Source: CAD feature listing. Evaluate the final solid. Frame: model axes, mm. A direction names the side the tool comes from. Give positions to 0.01 mm unless a question says otherwise; leave off trailing zeros. Order: outer loops, then holes, each group sorted by start corner. A loop starts at its lowest first (then second) coordinate and runs counter-clockwise, first axis right, second up.
1) Section B-B, the plane x = -20. Return loops of the section in (y, z), plus the area to 3 significant figures.
2) Section C-C, the plane y = 21. Return loops of the section in (x, z).
3) Section A-A, the plane z = 0. Return loops of the section in (x, y), plus the area to 3 significant figures.
4) Material intervals for line 1 (X direction, y = 65, z = 25.5); line 2 (Z direction, x = -20, y = 23); line 3 (Y direction, x = -32, z = -27) (3 decimals), sorted ascending.
5) First-contact query: P1, Ø10, axis at y = 13.5, z = 15.5, coming from the +X side; P2, Ø7, axis at x = 30.5, z = 2, coming from the +Y side; P3, Ø20.5, axis at x = 35, z = 0, coming from the +Y side. Flat tips, straight axial feed; report the tip coordinate or a pass-through.
6) Access query for faces 5 (the face through (5, 25, 0)), 6 (the face through (-33, 33, 18)), 7 (the face through (-30, 35, -24)). Directions: +Z, -Z, +X, -X, +Y, -Y. A direction counts if a zero-diameter tool reaches every point of the face in a straight line with its end or side. Return the directions, or none.
7) Section D-D, the plane x = 37.5. Return loops of the section in (y, z), plus the area to 3 significant figures.
8) Draft query along X for faces 1 (the face through (-37, 81, 24)), 2 (the face through (0, 0, 0)), 3 (the face through (-15.46, 68, -24.08)), 4 (the face through (-27.493, 20.28, -0.33)). Return one class per face: released by +X, released by -X, zero draft, split by the parting line, or undercut.
```python
from build123d import *

# Parameters (mm, degrees)
SKETCH1_R           = 10
BOSS_EXTRUDE1_DEPTH = 30
BOSS_EXTRUDE3_DEPTH = 8
SKETCH4_R           = 9
CUT_EXTRUDE5_DEPTH  = 8
SKETCH7_W           = 36
SKETCH7_H           = 64.778485803
CUT_EXTRUDE6_DEPTH  = 41
SKETCH8_W           = 30
SKETCH8_H           = 36
BOSS_EXTRUDE5_DEPTH = 15
SKETCH9_R           = 7.5
CUT_EXTRUDE8_DEPTH  = 41


with BuildPart() as part:
    # Sketch1 → Boss-Extrude1 (new body, symmetric)
    with BuildSketch(Plane.XY):
        with BuildLine():
            Line((-35, 25), (-35, 0))
            Line((-35, 0), (35, 0))
            Line((35, 0), (35, 12))
            Line((35, 12), (15, 12))
            Line((15, 12), (15, 25))
            Line((15, 25), (-5, 25))
            Line((-5, 25), (-5, 40))
            Line((-5, 40), (-5, 65))
            ThreePointArc((-5, 65), (-37.247448714, 80.811388301), (-30, 45.635083269))
            Line((-30, 45.635083269), (-30, 40))
            Line((-30, 40), (-30, 25))
            Line((-30, 25), (-35, 25))
        make_face()
        with Locations((-25, 65)):
            Circle(SKETCH1_R, mode=Mode.SUBTRACT)
    extrude(amount=BOSS_EXTRUDE1_DEPTH, both=True)

    # Sketch3 → Boss-Extrude3 (add)
    with BuildSketch(Plane(origin=(0, 12, 0), x_dir=(1, 0, 0), z_dir=(0, 1, 0))):
        with BuildLine():
            Line((15, 30), (35, 30))
            ThreePointArc((35, 30), (65, 0), (35, -30))
            Line((35, -30), (15, -30))
            Line((15, -30), (15, 30))
        make_face()
    extrude(amount=-BOSS_EXTRUDE3_DEPTH)

    # Sketch4 → Cut-Extrude5 (cut)
    with BuildSketch(Plane(origin=(0, 12, 0), x_dir=(1, 0, 0), z_dir=(0, 1, 0))):
        with Locations((35, 0)):
            Circle(SKETCH4_R)
    extrude(amount=-CUT_EXTRUDE5_DEPTH, mode=Mode.SUBTRACT)

    # Sketch7 → Cut-Extrude6 (cut, through all)
    with BuildSketch(Plane(origin=(-5, 0, 0), x_dir=(0, 0, -1), z_dir=(1, 0, 0))):
        with Locations((0, 72.389242902)):
            Rectangle(SKETCH7_W, SKETCH7_H)
    extrude(amount=-CUT_EXTRUDE6_DEPTH, mode=Mode.SUBTRACT)

    # Sketch8 → Boss-Extrude5 (add)
    with BuildSketch(Plane(origin=(0, 40, 0), x_dir=(1, 0, 0), z_dir=(0, 1, 0))):
        with Locations((-20, 0)):
            Rectangle(SKETCH8_W, SKETCH8_H)
    extrude(amount=-BOSS_EXTRUDE5_DEPTH)

    # Sketch9 → Cut-Extrude8 (cut, through all)
    with BuildSketch(Plane(origin=(0, 40, 0), x_dir=(1, 0, 0), z_dir=(0, 1, 0))):
        with Locations((-20, 0)):
            Circle(SKETCH9_R)
    extrude(amount=-CUT_EXTRUDE8_DEPTH, mode=Mode.SUBTRACT)


solid = part.part
```
From the geometry:
1. outline: (0, -30) - (56.34, -30) - (56.34, -18) - (40, -18) - (40, -7.5) - (0, -7.5) - close; (0, 7.5) - (40, 7.5) - (40, 18) - (56.34, 18) - (56.34, 30) - (0, 30) - close; (73.66, -30) - (84.36, -30) - (84.36, -18) - (73.66, -18) - close; (73.66, 18) - (84.36, 18) - (84.36, 30) - (73.66, 30) - close
1. area: 2,450 mm2
2. outline: (-35, -30) - (15, -30) - (15, 30) - (-35, 30) - close; hole circle Ø15 at (-20, 0)
3. outline: (-35, 0) - (-27.5, 0) - (-27.5, 40) - (-35, 40) - close; (-12.5, 0) - (35, 0) - (35, 4) - (26, 4) - (26, 12) - (15, 12) - (15, 25) - (-5, 25) - (-5, 40) - (-12.5, 40) - close; (44, 4) - (65, 4) - (65, 12) - (44, 12) - close
3. area: 1,440 mm2
4. line 1: x = -45 to -35, -15 to -5
4. line 2: z = -30 to -7.5, 7.5 to 30
4. line 3: y = 0 to 25, 46.265 to 57.859, 72.141 to 83.735
5. P1: stops at x = 63.02
5. P2: stops at y = 4
5. P3: stops at y = 12
6. face 5: +Z, -Z, +X, +Y
6. face 6: +Z, -X
6. face 7: -Z, -X
7. outline: (4, -29.9) - (12, -29.9) - (12, -8.65) - (4, -8.65) - close; (4, 8.65) - (12, 8.65) - (12, 29.9) - (4, 29.9) - close
7. area: 340 mm2
8. face 1: split by the parting line
8. face 2: zero draft
8. face 3: undercut
8. face 4: undercut
